```python
from build123d import *

# Parameters (mm, degrees)
ESQUISSE1_W             = 190
ESQUISSE1_H             = 10
ESQUISSE1_R             = 1.6
BOSS_EXTRU_1_DEPTH      = 2
ESQUISSE2_W             = 2
ESQUISSE2_H             = 10
BOSS_EXTRU_2_DEPTH      = 115
CONG_1_R                = 2
ENL_V_MAT_EXTRU_1_REACH = 226.029
ESQUISSE3_R             = 1.6


with BuildPart() as part:
    # Esquisse1 → Boss.-Extru.1 (new body)
    with BuildSketch(Plane.XY):
        with Locations((95, 5)):
            Rectangle(ESQUISSE1_W, ESQUISSE1_H)
        with Locations((5, 5)):
            Circle(ESQUISSE1_R, mode=Mode.SUBTRACT)
        with Locations((13, 5)):
            Circle(ESQUISSE1_R, mode=Mode.SUBTRACT)
        with Locations((21, 5)):
            Circle(ESQUISSE1_R, mode=Mode.SUBTRACT)
    extrude(amount=BOSS_EXTRU_1_DEPTH)

    # Esquisse2 → Boss.-Extru.2 (add)
    with BuildSketch(Plane.XY):
        with Locations((191, 5)):
            Rectangle(ESQUISSE2_W, ESQUISSE2_H)
    extrude(amount=BOSS_EXTRU_2_DEPTH)

    # Congé1
    cong_1_edges = [part.edges().sort_by_distance(p)[0] for p in [
        (192, 5, 0),
    ]]
    fillet(cong_1_edges, radius=CONG_1_R)

    # Esquisse3 → Enlèv. mat.-Extru.1 (cut, up to next)
    with BuildSketch(Plane(origin=(192, 0, 0), x_dir=(0, 0, -1), z_dir=(1, 0, 0)), mode=Mode.PRIVATE) as enl_v_mat_extru_1_sk1:
        with Locations((-91, 5.5)):
            Circle(ESQUISSE3_R)
    enl_v_mat_extru_1_tool1 = extrude(enl_v_mat_extru_1_sk1.sketch, amount=-ENL_V_MAT_EXTRU_1_REACH, mode=Mode.PRIVATE) & part.part
    # Esquisse3 → Enlèv. mat.-Extru.1 (cut, up to next)
    with BuildSketch(Plane(origin=(192, 0, 0), x_dir=(0, 0, -1), z_dir=(1, 0, 0)), mode=Mode.PRIVATE) as enl_v_mat_extru_1_sk2:
        with Locations((-26, 5.5)):
            Circle(ESQUISSE3_R)
    enl_v_mat_extru_1_tool2 = extrude(enl_v_mat_extru_1_sk2.sketch, amount=-ENL_V_MAT_EXTRU_1_REACH, mode=Mode.PRIVATE) & part.part
    add(enl_v_mat_extru_1_tool1.solids().sort_by_distance((192, 5.5, 91))[0], mode=Mode.SUBTRACT)
    add(enl_v_mat_extru_1_tool2.solids().sort_by_distance((192, 5.5, 26))[0], mode=Mode.SUBTRACT)


solid = part.part
```
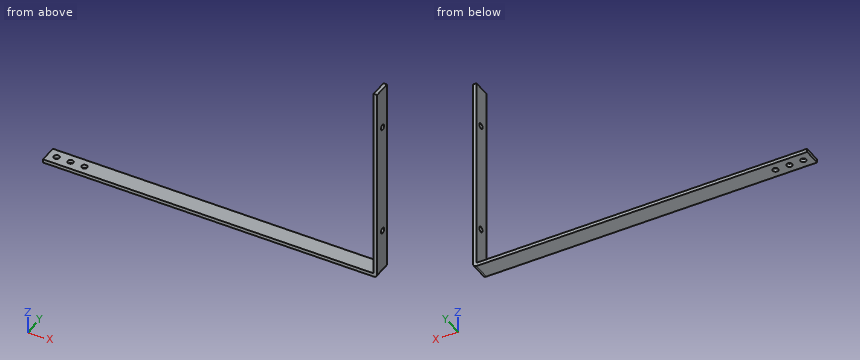
The listing builds one solid part. Answer for the finished solid, in the listing's coordinates (mm). Coordinates: 2 decimals unless noted, no trailing zeros. Order: outer loops, then holes, each group sorted by start corner. A loop starts at its lowest first (then second) coordinate and runs counter-clockwise, first axis right, second up. Notation, with made-up numbers: M 8.25,-30.75 L 14.25,-30.75 A34 cw 14.25,1.25 Z; hole C -25,21.25 d4. An arc over 180 degrees is marked long. Answer as a JSON object with one key per item and string values. Group by question number.
1. Flat-ended cylindrical pins translate along their axes: P1, Ø2, axis at y = 4.5, z = 81, coming from the -X side; P2, Ø3.5, axis at x = 5, y = 5, coming from the +Z side. Find the tip coordinate at first contact, or state that the pin passes through.
2. Section B-B on x = 57 is taken. Write down the section's boundary in (y, z), then the cut area to 3 significant figures.
3. Straight lines are drawn through the part: line 1 (Y direction, x = 21, z = 0.5); line 2 (Y direction, x = 191, z = 91); line 3 (X direction, y = 7.75, z = 16.5). For each, find the intervals that lie inside material, in ascending order.
4. Section A-A on z = 56.5 is taken. Write down the section's boundary in (x, y).
Values follow:
{
 "1": {"P1": "x = 190", "P2": "z = 2"},
 "2": {"outline": "M 0,0 L 10,0 L 10,2 L 0,2 Z", "area": "20.0 mm2"},
 "3": {"line 1": "0 to 3.4, 6.6 to 10", "line 2": "0 to 3.9, 7.1 to 10", "line 3": "190 to 192"},
 "4": {"outline": "M 190,0 L 192,0 L 192,10 L 190,10 Z"}
}
